```python
from build123d import *

# Parameters (mm, degrees)
BOSS_EXTRUDE1_DEPTH = 45
SKETCH2_W           = 35
SKETCH2_H           = 45
BOSS_EXTRUDE2_DEPTH = 5
SKETCH3_R           = 2.2
CUT_EXTRUDE1_DEPTH  = 5


with BuildPart() as part:
    # Sketch1 → Boss-Extrude1 (new body)
    with BuildSketch(Plane(origin=(0, 0, 0), x_dir=(1, 0, 0), z_dir=(0, 1, 0))):
        Polygon((150, 50), (0, 0), (59.974081308, 0), (150, 30), align=None)
    extrude(amount=BOSS_EXTRUDE1_DEPTH)

    # Sketch2 → Boss-Extrude2 (add)
    with BuildSketch(Plane(origin=(150, 0, 0), x_dir=(0, 0, -1), z_dir=(1, 0, 0))):
        with Locations((47.5, 22.5)):
            Rectangle(SKETCH2_W, SKETCH2_H)
    extrude(amount=-BOSS_EXTRUDE2_DEPTH)

    # Sketch3 → Cut-Extrude1 (cut)
    with BuildSketch(Plane.ZY.offset(-145)):
        with Locations((-56.666666667, 33.75)):
            Circle(SKETCH3_R)
        with Locations((-56.666666667, 11.25)):
            Circle(SKETCH3_R)
    extrude(amount=-CUT_EXTRUDE1_DEPTH, mode=Mode.SUBTRACT)


solid = part.part
```
Can you work these out from the model? Positions are in its coordinate system, mm. A direction names the side the tool comes from. Give positions to 0.01 mm unless a question says otherwise; leave off trailing zeros. Order: outer loops, then holes, each group sorted by start corner. A loop starts at its lowest first (then second) coordinate and runs counter-clockwise, first axis right, second up. Notation, with made-up numbers: (-4.5, 19) - (31.5, 19) arc R8 cw to (31.5, 26) - close; hole circle Ø4 at (-0.5, 24.5). An arc over 180 degrees is marked (long way). Use a Markdown table: item, result. Add a question column.
Q1. If we mould it in two halves opening along Y, with no side actions, what happens to faces 3 (the flat face through (91, 0, -21)), 4 (the cylindrical face through (147.465, 32.907, -54.634)), 5 (the flat face through (30, 22, 0)), 6 (the cylindrical face through (147.46, 11.91, -54.57))? For each: released by +Y, released by -Y, zero draft, split by the parting line, or undercut.
Q2. Please list where these lines run through material, in increasing order: line 1 along X through (y, z) = (41.5, -59); line 2 along Z through (x, y) = (49.5, 29); line 3 along Z through (x, y) = (102, 35).
Q3. If we section it at A-A on y = 11.25: Write out the boundary of the cut face in (x, z), plus the area to 3 significant figures.
Q4. If we section it at C-C on x = 29: Write out the boundary of the cut face in (y, z), plus the area to 3 significant figures.
Q5. On a 3-axis mill with a long thin cutter (end or side, diameter ignored), from which of +Z, -Z, +X, -X, +Y, -Y can I reach the whole of each face in a straight line? I mean faces 1 (the flat face through (148, 22, -65)), 2 (the flat face through (145, 23, -57)). Say none if no direction works.
Q6. I'm going to push flat-ended pins straight in: pin 1 (3.5 mm diameter, centred on y = 33.75, z = -56.67, fed in from -X); pin 2 (1 mm diameter, centred on x = 62, y = 8, fed in from -Z); pin 3 (1 mm diameter, centred on x = 32, y = 22, fed in from -Z); pin 4 (8 mm diameter, centred on x = 85, y = 35, fed in from +Z). Where does each tip first touch, or does it pass through?
Q7. If we section it at B-B on y = 21: Write out the boundary of the cut face in (x, z), plus the area to 3 significant figures.
Q8. If we section it at D-D on z = -4: Write out the boundary of the cut face in (x, y).
Answers follow:
| question | item | result |
|---|---|---|
| 1 | face 3 | released by -Y |
| 1 | face 4 | undercut |
| 1 | face 5 | zero draft |
| 1 | face 6 | undercut |
| 2 | line 1 | x = 145 to 150 |
| 2 | line 2 | z = -16.5 to 0 |
| 2 | line 3 | z = -34 to -14 |
| 3 | outline | (0, 0) - (145, -48.33) - (145, -54.47) - (150, -54.47) - (150, -30) - (59.97, 0) - close; (145, -65) - (150, -65) - (150, -58.87) - (145, -58.87) - close |
| 3 | area | 2,460 mm^2 |
| 4 | outline | (0, -9.67) - (45, -9.67) - (45, 0) - (0, 0) - close |
| 4 | area | 435 mm^2 |
| 5 | face 1 | -Z, +X, -X, +Y, -Y |
| 5 | face 2 | -Z, -X, +Y, -Y |
| 6 | pin 1 | passes through |
| 6 | pin 2 | stops at z = -20.83 |
| 6 | pin 3 | stops at z = -10.83 |
| 6 | pin 4 | stops at z = -7.01 |
| 7 | outline | (0, 0) - (145, -48.33) - (145, -65) - (150, -65) - (150, -30) - (59.97, 0) - close |
| 7 | area | 2,480 mm^2 |
| 8 | outline | (12, 0) - (71.98, 0) - (71.98, 45) - (12, 45) - close |
